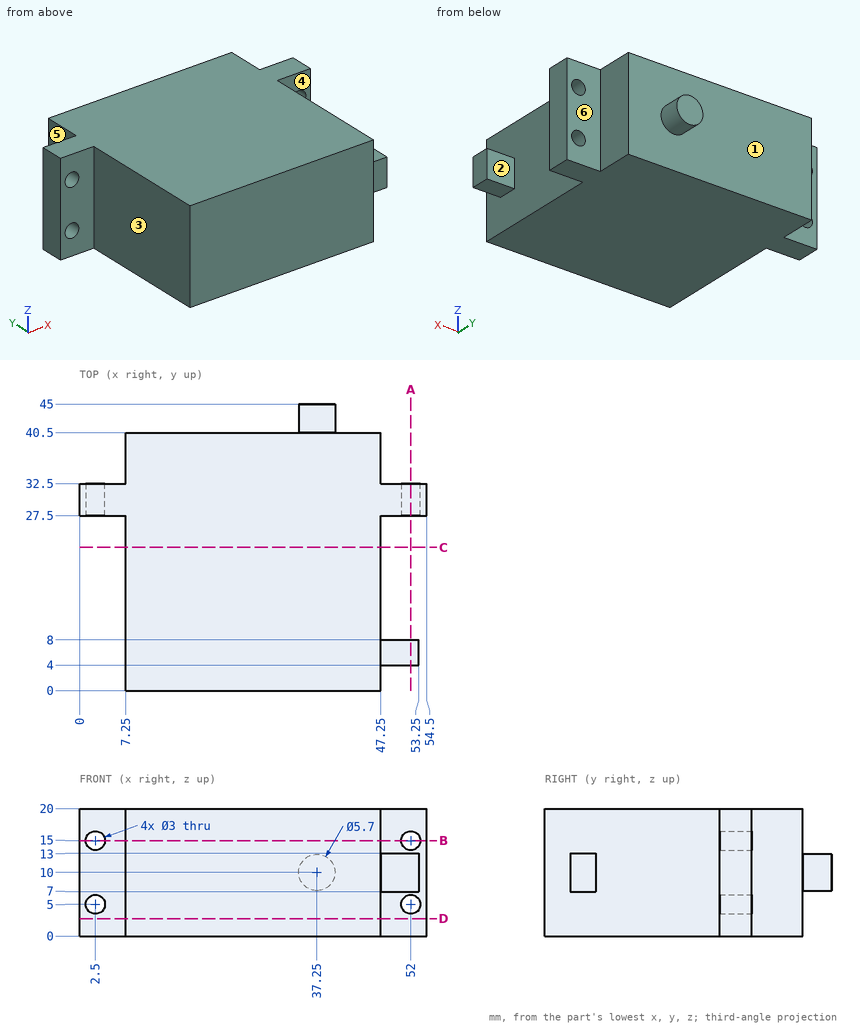
Design review of the part shown in the three views and the two pictorial views. Dimensions are in mm from the part's minimum x, y and z. A direction names the side the tool comes from. Coordinates: 2 decimals unless noted, no trailing zeros. Loops run counter-clockwise (first coordinate to the right, second up) from the corner with the lowest first, then second, coordinate; pieces in that order, holes last. Notation, with made-up numbers: (2, -9.5) - (51, -9.5) arc R10 cw to (51, 7.5) - close; hole circle Ø3 at (11.25, 84.25). An arc over 180 degrees is marked (long way). Use a Markdown table: item, result. Add a question column.
Item 1: Insertion check: pin 1 Ø5 at (x, z) = (49, 11) entering from -Y; pin 2 Ø3.5 at (x, z) = (4.5, 10.5) entering from +Y; pin 3 Ø1.5 at (x, z) = (47.5, 4) entering from +Y; pin 4 Ø2 at (y, z) = (8, 13) entering from +X. Each pin has a flat end and moves straight along its axis. Give the tip position at first contact, or say it passes through.
Item 2: We need section B-B (z = 15). Give the boundary of the cut face in (x, y), and give its area (3 significant figures).
Item 3: Tool access review of the marked faces 4, 5 and 6: name each direction out of +Z, -Z, +X, -X, +Y, -Y from which nothing blocks a thin tool from reaching the whole face with its end or side.
Item 4: We need section A-A (x = 52). Give the boundary of the cut face in (y, z), and give its area (3 significant figures).
Item 5: Mouldability with a two-part tool opening along Y and no side actions: class the marked faces 1, 2 and 3 as pulls with the +Y half, pulls with the -Y half, needs draft (parallel to the pull), parting line crosses it, or undercut.
Item 6: We need section D-D (z = 2.75). Give the boundary of the cut face in (x, y).
Item 7: For line 1 (Z direction, x = 2.5, y = 31.4); line 2 (X direction, y = 31, z = 6); line 3 (X direction, y = 26.5, z = 5.75), list the stretches that pass through material, from the lowest coordinate up.
Item 8: We need section C-C (y = 22.5). Give the boundary of the cut face in (x, z).
Results list:
| question | item | result |
|---|---|---|
| 1 | pin 1 | stops at y = 0 |
| 1 | pin 2 | stops at y = 32.5 |
| 1 | pin 3 | stops at y = 40.5 |
| 1 | pin 4 | stops at x = 53.25 |
| 2 | outline | (0, 27.5) - (1, 27.5) - (1, 32.5) - (0, 32.5) - close; (4, 27.5) - (7.25, 27.5) - (7.25, 0) - (47.25, 0) - (47.25, 27.5) - (50.5, 27.5) - (50.5, 32.5) - (47.25, 32.5) - (47.25, 40.5) - (7.25, 40.5) - (7.25, 32.5) - (4, 32.5) - close; (53.5, 27.5) - (54.5, 27.5) - (54.5, 32.5) - (53.5, 32.5) - close |
| 2 | area | 1,660 mm^2 |
| 3 | face 4 | +Z, -Z, +X |
| 3 | face 5 | +Z, -Z, -X, +Y |
| 3 | face 6 | +Z, -Z, +X, +Y |
| 4 | outline | (4, 7) - (8, 7) - (8, 13) - (4, 13) - close; (27.5, 0) - (32.5, 0) - (32.5, 3.5) - (27.5, 3.5) - close; (27.5, 6.5) - (32.5, 6.5) - (32.5, 13.5) - (27.5, 13.5) - close; (27.5, 16.5) - (32.5, 16.5) - (32.5, 20) - (27.5, 20) - close |
| 4 | area | 94.0 mm^2 |
| 5 | face 1 | pulls with the +Y half |
| 5 | face 2 | undercut |
| 5 | face 3 | needs draft |
| 6 | outline | (0, 27.5) - (7.25, 27.5) - (7.25, 0) - (47.25, 0) - (47.25, 27.5) - (54.5, 27.5) - (54.5, 32.5) - (47.25, 32.5) - (47.25, 40.5) - (7.25, 40.5) - (7.25, 32.5) - (0, 32.5) - close |
| 7 | line 1 | z = 0 to 3.5, 6.5 to 13.5, 16.5 to 20 |
| 7 | line 2 | x = 0 to 1.38, 3.62 to 50.88, 53.12 to 54.5 |
| 7 | line 3 | x = 7.25 to 47.25 |
| 8 | outline | (7.25, 0) - (47.25, 0) - (47.25, 20) - (7.25, 20) - close |
